```python
from build123d import *

# Parameters (mm, degrees)
BOSS_EXTRUDE1_DEPTH = 6
CUT_EXTRUDE1_DEPTH  = 59.057322490699136
BOSS_EXTRUDE2_DEPTH = 32
BOSS_EXTRUDE3_DEPTH = 0.2
BOSS_EXTRUDE4_DEPTH = 15
BOSS_EXTRUDE5_DEPTH = 6
CUT_EXTRUDE2_DEPTH  = 70.12779972477816
SKETCH8_R           = 1.5000000000000042
SKETCH8_R_2         = 1.5000000000000018
CUT_EXTRUDE3_DEPTH  = 70.12779972477817
SKETCH9_W           = 2.49999999999999
SKETCH9_H           = 5.999999999999993
BOSS_EXTRUDE6_DEPTH = 15
CUT_EXTRUDE4_DEPTH  = 3
BOSS_EXTRUDE7_DEPTH = 3
FILLET1_R           = 3


with BuildPart() as part:
    # Sketch1 → Boss-Extrude1 (new body)
    with BuildSketch(Plane.XY):
        Polygon((-25, 22.000000000000007), (1.7101007166283717, 11.425886468780801), (19.33568195921926, -36.99999999999998), (2.500000000000002, -36.999999999999986), (2.500000000000002, -21.999999999999986), (-25.000000000000004, -21.99999999999999), align=None)
    extrude(amount=BOSS_EXTRUDE1_DEPTH)

    # Sketch2 → Cut-Extrude1 (cut, through all)
    with BuildSketch(Plane.ZY.offset(25.000000000000004)):
        Polygon((-4.44e-15, 18.499999999999993), (5.999999999999988, 12.499999999999988), (5.999999999999991, 22.000000000000007), (0, 22.000000000000004), align=None)
    extrude(amount=-CUT_EXTRUDE1_DEPTH, mode=Mode.SUBTRACT)

    # Sketch3 → Boss-Extrude2 (add)
    with BuildSketch(Plane(origin=(0, 0, 0), x_dir=(-1, 0, 0), z_dir=(0, 0, -1))):
        Polygon((-1.7101007166283715, 11.425886468780803), (-19.33568195921926, -36.99999999999998), (-2.500000000000002, -36.999999999999986), (-2.500000000000002, -21.999999999999986), (0, -21.999999999999986), (-9.2e-16, 1.3500000000000014), (-0.2, 1.3499999999999996), (-0.2, 12.023711860403642), align=None)
    extrude(amount=BOSS_EXTRUDE2_DEPTH)

    # Sketch4 → Boss-Extrude3 (add)
    with BuildSketch(Plane.ZY.offset(-0.2)):
        with BuildLine():
            Line((-32, 12.02371186040364), (-32, 1.3499999999999996))
            Line((-32, 1.3499999999999996), (-19.46806862677186, 1.3499999999999996))
            ThreePointArc((-19.468068626771874, 1.3499999999999552), (-23.244240803514778, 6.058100110538283), (-22.32927664622476, 12.023711860403747))
            Line((-22.32927664622472, 12.02371186040364), (-32, 12.02371186040364))
        make_face()
        with BuildLine():
            ThreePointArc((-8.499999999999993, 7.999999999999998), (-9.586712438195622, 4.111588672786104), (-12.531931373228087, 1.3499999999999694))
            Line((-12.53193137322809, 1.3499999999999999), (0, 1.3499999999999999))
            Line((0, 1.3499999999999979), (0, 12.023711860403642))
            Line((0, 12.02371186040364), (-9.670723353775251, 12.02371186040364))
            ThreePointArc((-9.67072335377522, 12.023711860403733), (-8.798626004480603, 10.09528341201306), (-8.499999999999993, 8))
        make_face()
    extrude(amount=BOSS_EXTRUDE3_DEPTH)

    # Sketch5 → Boss-Extrude4 (add)
    with BuildSketch(Plane.XZ.offset(21.999999999999986)):
        with BuildLine():
            Line((-1.86e-15, 0), (-1.86e-15, -6.333801512904159))
            ThreePointArc((-1.1013e-13, -6.333801512904192), (1.8581867686024491, -9.836881046371968), (2.4999999999999964, -13.750000014767066))
            Line((2.4999999999999973, -13.750000014767064), (2.4999999999999973, 6.000000000000006))
            Line((2.4999999999999973, 6.000000000000006), (-1.8e-15, 6))
            Line((-1.8e-15, 6), (-1.86e-15, 0))
        make_face()
        with BuildLine():
            Line((-1.86e-15, -21.166198487095418), (-1.86e-15, -32))
            Line((-1.78e-15, -32), (2.4999999999999973, -32))
            Line((2.4999999999999973, -32), (2.4999999999999973, -13.750000014767064))
            ThreePointArc((2.4999999999999964, -13.750000014767066), (1.8581867638853513, -17.6631189676212), (1.4744e-13, -21.166198487095464))
        make_face()
    extrude(amount=BOSS_EXTRUDE4_DEPTH)

    # Sketch6 → Boss-Extrude5 (add)
    with BuildSketch(Plane(origin=(2.66e-15, 0, -32), x_dir=(-1, 0, -8e-17), z_dir=(8e-17, 0, -1))):
        Polygon((25, 22.000000000000007), (-1.7101007166283717, 11.425886468780801), (-19.33568195921926, -36.99999999999998), (-2.500000000000002, -36.999999999999986), (-2.500000000000002, -21.999999999999986), (25.000000000000004, -21.99999999999999), align=None)
    extrude(amount=BOSS_EXTRUDE5_DEPTH)

    # Sketch7 → Cut-Extrude2 (cut, through all)
    with BuildSketch(Plane.ZY.offset(25.000000000000004)):
        Polygon((-38.00000000000001, 22.000000000000004), (-32, 22.000000000000004), (-32, 18.499999999999982), (-38.00000000000001, 12.49999999999995), align=None)
    extrude(amount=-CUT_EXTRUDE2_DEPTH, mode=Mode.SUBTRACT)

    # Sketch8 → Cut-Extrude3 (cut, through all)
    with BuildSketch(Plane.ZY.offset(25.000000000000004)):
        with Locations((-34.99999999999999, 8.428932188134494)):
            Circle(SKETCH8_R)
        with Locations((-34.99999999999999, -17.000000000000004)):
            Circle(SKETCH8_R)
        with Locations((3.0000000000000027, -16.99999999999999)):
            Circle(SKETCH8_R_2)
        with Locations((2.9999999999999956, 8.428932188134505)):
            Circle(SKETCH8_R_2)
    extrude(amount=-CUT_EXTRUDE3_DEPTH, mode=Mode.SUBTRACT)

    # Sketch9 → Boss-Extrude6 (add)
    with BuildSketch(Plane.XZ.offset(36.999999999999986)):
        with Locations((1.249999999999995, -35)):
            Rectangle(SKETCH9_W, SKETCH9_H)
    extrude(amount=-BOSS_EXTRUDE6_DEPTH)

    # Sketch10 → Cut-Extrude4 (cut)
    with BuildSketch(Plane(origin=(5.182266059796382, 1.8861905918139033, 0), x_dir=(0, 0, -1), z_dir=(0.939692620785907, 0.34202014332567265, 0))):
        Polygon((37.99999999999999, -41.38181968407034), (37.99999999999999, -17.381819684070333), (-5.999999999999991, -17.381819684070337), (-6.00000000000001, -41.38181968407034), align=None)
    extrude(amount=-CUT_EXTRUDE4_DEPTH, mode=Mode.SUBTRACT)

    # Sketch11 → Boss-Extrude7 (add)
    # profile 1 of 2: a face of its own
    with BuildSketch(Plane(origin=(2.363188197438662, 0.8601301618368854, 0), x_dir=(0, 0, -1), z_dir=(0.939692620785907, 0.3420201433256727, 0))):
        with BuildLine():
            ThreePointArc((0.499999999999996, -19.00635353175345), (0.39856604189581324, -18.16984360421368), (0.10014350921565462, -17.38181968407036))
            Line((0.10014350921566262, -17.38181968407034), (-5.999999999999993, -17.38181968407034))
            Line((-5.999999999999991, -17.38181968407034), (-5.999999999999994, -20.809129169485423))
            ThreePointArc((-6.000000000000014, -20.809129169485427), (-2.0645856533065285, -22.379037922561462), (0.499999999999996, -19.00635353175345))
        make_face()
        with BuildLine():
            add(Edge.make_bspline(
                [(-3.000000000000003, -17.410086873039575), (-5.598076211353321, -17.410086873039575), (-4.299038105676663, -19.804486861110384), (-3.0000000000000044, -22.198886849181193), (-1.7009618943233444, -19.804486861110384), (-0.4019237886466831, -17.410086873039578), (-3.0000000000000027, -17.410086873039575)],
                knots=[0, 0, 0, 2.0943951023931953, 2.0943951023931953, 4.1887902047863905, 4.1887902047863905, 6.283185307179586, 6.283185307179586, 6.283185307179586], degree=2, weights=[1, 0.5000000000000001, 1, 0.5000000000000001, 1, 0.5000000000000001, 1]))
        make_face(mode=Mode.SUBTRACT)
    # profile 2 of 2: a face of its own
    with BuildSketch(Plane(origin=(2.363188197438662, 0.8601301618368854, 0), x_dir=(0, 0, -1), z_dir=(0.939692620785907, 0.3420201433256727, 0))):
        with BuildLine():
            Line((37.99999999999999, -20.809129169485587), (37.99999999999999, -17.381819684070337))
            Line((37.99999999999999, -17.381819684070337), (31.899856490784423, -17.381819684070337))
            ThreePointArc((31.899856490784394, -17.38181968407025), (33.28561388310159, -22.057727032684816), (37.99999999999992, -20.80912916948557))
        make_face()
        with BuildLine():
            add(Edge.make_bspline(
                [(34.999999999999986, -17.41008687303959), (32.40192378864666, -17.41008687303959), (33.70096189432332, -19.8044868611104), (34.999999999999986, -22.198886849181218), (36.299038105676644, -19.804486861110405), (37.59807621135331, -17.410086873039592), (34.999999999999986, -17.41008687303959)],
                knots=[0, 0, 0, 2.0943951023931953, 2.0943951023931953, 4.1887902047863905, 4.1887902047863905, 6.283185307179586, 6.283185307179586, 6.283185307179586], degree=2, weights=[1, 0.5000000000000001, 1, 0.5000000000000001, 1, 0.5000000000000001, 1]))
        make_face(mode=Mode.SUBTRACT)
    extrude(amount=BOSS_EXTRUDE7_DEPTH)

    # Fillet1
    fillet1_edges = [part.edges().sort_by_distance(p)[0] for p in [
        (9.717659588224263, -14.960407316126739, -0.10014350921565796),
        (9.717659588224242, -14.960407316126686, -31.89985649078441),
    ]]
    fillet(fillet1_edges, radius=FILLET1_R)


solid = part.part
```
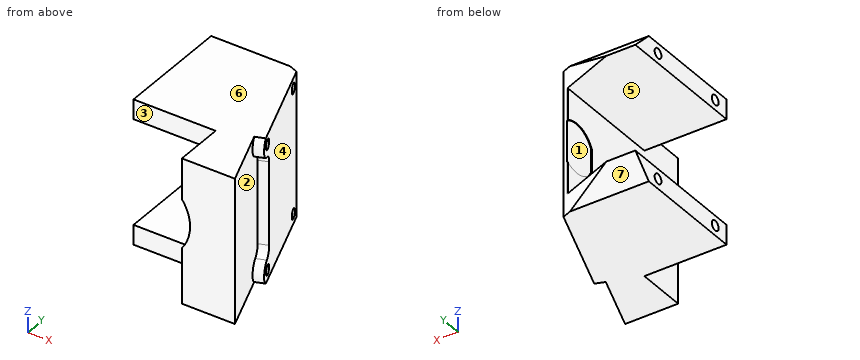
CAD build for the part. Positions are in the model's coordinates, mm. Face numbers are marked on the shaded views. A direction names the side the tool comes from. Round coordinates to 2 decimals unless told otherwise and drop trailing zeros. Write each loop counter-clockwise with the first axis right and the second up, starting at its lowest first coordinate (ties: lowest second). Pieces come first, ordered by that corner, then holes. Notation, with made-up numbers: (15.25, -10) - (69.25, -10) arc R13 cw to (69.25, 11) - close; hole circle Ø6 at (89.25, 73). An arc over 180 degrees is marked (long way). Write item = value, one per line. Start each with the question number.
Q1. Band-saw the part on D-D (z = -14.5). Give the cut face in (x, y).
Q2. Band-saw the part on B-B (y = -31). Give the cut face in (x, z).
Q3. Mould opens along Z. For the marked faces 4, 5, 6 and 7 say: pulls with the +Z half, pulls with the -Z half, needs draft (parallel to the pull), parting line crosses it, or undercut.
Q4. Drop flat-ended pins along their axis: pin 1 (5.5 mm diameter, centred on y = 5.5, z = -13, fed in from -X); pin 2 (12 mm diameter, centred on y = -14.5, z = -33.5, fed in from +X); pin 3 (2 mm diameter, centred on y = -3.5, z = -21, fed in from +X); pin 4 (8 mm diameter, centred on x = -6.5, y = -24.5, fed in from +Z). Give the stop position or say it passes through.
Q5. Band-saw the part on C-C (z = 3). Count the separate pieces of the cut face and the enclosed holes in it, then the cut area to 3 significant figures.
Q6. Probe L1, parallel to Z at x = -23, y = 1; L2, parallel to Y at x = -8, z = 3; L3, parallel to Y at x = -7, z = -35. List the from-to ranges inside material, lowest first. Write a range as from..to.
Q7. Band-saw the part on A-A (x = -14). Give the cut face in (y, z).
Q8. Which spindle directions (+Z, -Z, +X, -X, +Y, -Y) get a long thin tool onto all of the face, cutting with end or side? Do the marked faces 1, 2 and 3. Say none if no direction does.
Answers below:
q1.outline = (0, -22) - (2.48, -22) - (2.48, -37) - (16.14, -37) - (8.31, -15.47) - (11.13, -14.45) - (1.71, 11.43) - (0.2, 12.02) - (0.2, 1.35) - (0, 1.35) - close
q2.outline = (0, -38) - (13.96, -38) - (13.96, 6) - (0, 6) - (0, -6.33) arc R12.25 cw to (0, -21.17) - close
q3.face_4 = needs draft
q3.face_5 = undercut
q3.face_6 = pulls with the +Z half
q3.face_7 = pulls with the -Z half
q4.pin_1 = 0.2
q4.pin_2 = 12.88
q4.pin_3 = 7.51
q4.pin_4 = 6
q5.separate_pieces = 3
q5.enclosed_holes = 0
q5.area = 1,180 mm2
q6.L1 = -38..-32, 0..6
q6.L2 = -22..-18.5, -15.5..6.93, 9.93..15.27
q6.L3 = -22..-18.5, -15.5..6.93, 9.93..14.87
q7.outline = (-22, -38) - (12.5, -38) - (17.65, -32.85) - (17.65, -32) - (-22, -32) - close; (-22, 0) - (17.65, 0) - (17.65, 0.85) - (12.5, 6) - (-22, 6) - close; hole circle Ø3 at (-17, -35); hole circle Ø3 at (-17, 3); hole circle Ø3 at (8.43, -35); hole circle Ø3 at (8.43, 3)
q8.face_1 = -X
q8.face_2 = +X
q8.face_3 = +Z, -Z, -X, -Y
